Geometry check sheet. Reference: the model listing, model coordinates, mm. A direction names the side the tool comes from. Round coordinates to 2 decimals unless told otherwise and drop trailing zeros. Write each loop counter-clockwise with the first axis right and the second up, starting at its lowest first coordinate (ties: lowest second). Pieces come first, ordered by that corner, then holes. Notation, with made-up numbers: M 4,70 L 23,70 A20 cw 23,75 Z; hole C -11,69.25 d7. An arc over 180 degrees is marked long. One line per item, written item: value. Start each with the question number.
1. Section check D-D (z = 13.5). Record the boundary of the cut face in (x, y), and give its area (3 significant figures).
2. Scan lines: probe 1 along X at (y, z) = (-6, 27); probe 2 along X at (y, z) = (-19.5, 6); probe 3 along Z at (x, y) = (-12, 30). Record each from-to range of solid material in increasing order. Write a range as [from, to].
3. Depth check by flat-ended pin: P1, Ø1.5, axis at x = -10, z = 14.5, coming from the -Y side; P2, Ø1.5, axis at x = -10, z = 12.5, coming from the +Y side; P3, Ø6, axis at x = 0, z = 8, coming from the -Y side. Enter the tip coordinate at first touch or a pass-through.
4. Access from +Z, -Z, +X, -X, +Y, -Y to the whole of each face (thin tool, end or side, straight path). Record for faces 1 (the cylindrical face through (0.72, -15.54, 4.78)), 2 (the flat face through (-11, -2.4, 18)), 3 (the cylindrical face through (-4.845, 21.819, 7.888)), 4 (the flat face through (24, 0, 22)).
5. Release check for a two-part mould opening along Y. For faces 5 (the flat face through (7, -7, 37)), 6 (the cylindrical face through (-35.665, 1.57, 26.353)), 7 (the cylindrical face through (-32.192, 0.35, 29.605)) record: pulls with the +Y half, pulls with the -Y half, needs draft (parallel to the pull), parting line crosses it, or undercut.
6. Section check C-C (x = 26.5). Record the boundary of the cut face in (y, z).
7. Section check B-B (z = 24.5). Record the boundary of the cut face in (x, y), and give its area (3 significant figures).
8. Section check A-A (x = 0). Record the boundary of the cut face in (y, z), and give its area (3 significant figures).
from build123d import *

# Parameters (mm, degrees)
F0_R      = 35.7
F1_DEPTH  = 37
F3_R      = 35.7
F3_R_2    = 22.35
F4_DEPTH  = 16
F6_DEPTH  = 37.001
F7_R      = 7.95
F8_DEPTH  = 15
F12_D     = 6.6
F12_DEPTH = 35.7
F12_TIP   = 1.9828400428


with BuildPart() as f1:
    # F0 (on Top) → F1 (new body)
    with BuildSketch(Plane.XY):
        Circle(F0_R)
    extrude(amount=F1_DEPTH)

    # F3 (on face) → F4 (cut)
    with BuildSketch(Plane(origin=(0, 0, 0), x_dir=(1, 0, 0), z_dir=(0, 0, -1))):
        Circle(F3_R)
        Circle(F3_R_2, mode=Mode.SUBTRACT)
    extrude(amount=-F4_DEPTH, mode=Mode.SUBTRACT)

    # F5 (on face) → F6 (cut, through all)
    with BuildSketch(Plane(origin=(0, 0, 0), x_dir=(1, 0, 0), z_dir=(0, 0, -1))):
        with BuildLine():
            ThreePointArc((-9.191844211, -2.4), (-9.5, 0), (-9.191844211, 2.4))
            Line((-9.191844211, 2.4), (-12.1, 2.4))
            Line((-12.1, 2.4), (-12.1, -2.4))
            Line((-12.1, -2.4), (-9.191844211, -2.4))
        make_face()
        with BuildLine():
            Line((0, 2.4), (-9.191844211, 2.4))
            ThreePointArc((-9.191844211, 2.4), (-9.5, 0), (-9.191844211, -2.4))
            Line((-9.191844211, -2.4), (0, -2.4))
            Line((0, -2.4), (0, 2.4))
        make_face()
        with BuildLine():
            ThreePointArc((-9.191844211, -2.4), (1.2098512295, -9.4226461253), (9.5, 0))
            ThreePointArc((9.5, 0), (1.2098512295, 9.4226461253), (-9.191844211, 2.4))
            Line((-9.191844211, 2.4), (0, 2.4))
            Line((0, 2.4), (0, -2.4))
            Line((0, -2.4), (-9.191844211, -2.4))
        make_face()
    extrude(amount=-F6_DEPTH, mode=Mode.SUBTRACT)

    # F7 (on face) → F8 (cut)
    with BuildSketch(Plane.XY.offset(37)):
        with Locations((-24.25, 0)):
            Circle(F7_R)
        with Locations((24.25, 0)):
            Circle(F7_R)
    extrude(amount=-F8_DEPTH, mode=Mode.SUBTRACT)

    # F12
    with Locations(Plane.XZ.offset(35.7)):
        with Locations((0, 8)):
            Hole(F12_D / 2, depth=F12_DEPTH)
            with Locations((0, 0, -(F12_DEPTH + F12_TIP / 2))):  # 118° drill point
                Cone(0, F12_D / 2, F12_TIP, mode=Mode.SUBTRACT)


solid = f1.part
Result sheet:
1. outline: C 0,0 d44.7; hole M -12.1,-2.4 L -9.19,-2.4 A9.5 ccw long -9.19,2.4 L -12.1,2.4 Z
1. area: 1,270 mm2
2. probe 1: x = [-35.19, -29.47], [-19.03, -7.37], [7.37, 19.03], [29.47, 35.19]
2. probe 2: x = [-10.92, -2.62], [2.62, 10.92]
2. probe 3: z = [16, 37]
3. P1: stops at y = -20.35
3. P2: stops at y = 20.35
3. P3: stops at y = 9.01
4. face 1: -Y
4. face 2: +Z, -Z
4. face 3: -Z
4. face 4: +Z
5. face 5: needs draft
5. face 6: parting line crosses it
5. face 7: undercut
6. outline: M -23.92,16 L 23.92,16 L 23.92,37 L 7.62,37 L 7.62,22 L -7.62,22 L -7.62,37 L -23.92,37 Z
7. outline: C 0,0 d71.4; hole C -24.25,0 d15.9; hole M -12.1,-2.4 L -9.19,-2.4 A9.5 ccw long -9.19,2.4 L -12.1,2.4 Z; hole C 24.25,0 d15.9
7. area: 3,310 mm2
8. outline: M -35.7,16 L -22.35,16 L -22.35,11.3 L -9.5,11.3 L -9.5,37 L -35.7,37 Z; M -22.35,0 L -9.5,0 L -9.5,4.7 L -22.35,4.7 Z; M 9.5,0 L 22.35,0 L 22.35,16 L 35.7,16 L 35.7,37 L 9.5,37 Z
8. area: 1,430 mm2
